```python
from build123d import *

# Parameters (mm, degrees)
SKETCH1_W           = 42.2
SKETCH1_H           = 5
SKETCH1_H_2         = 20
SKETCH1_R           = 1.275
SKETCH1_R_2         = 13
BOSS_EXTRUDE3_DEPTH = 5
SKETCH1_3_W         = 42.2
SKETCH1_3_H         = 5
BOSS_EXTRUDE4_DEPTH = 50
CUT_EXTRUDE1_DEPTH  = 109.583838576
SKETCH3_R           = 2.5
CUT_EXTRUDE2_DEPTH  = 81.037803568
SKETCH5_W           = 82.2
SKETCH5_H           = 50
SKETCH5_R           = 2.5
CUT_EXTRUDE3_DEPTH  = 2


with BuildPart() as part:
    # Sketch1 → Boss-Extrude3 (new body)
    # profile 1 of 6: a face of its own
    with BuildSketch(Plane(origin=(0, 0, 0), x_dir=(1, 0, 0), z_dir=(0, 1, 0))):
        with Locations((0, 43.6)):
            Rectangle(SKETCH1_W, SKETCH1_H)
    # profile 2 of 6: a face of its own
    with BuildSketch(Plane(origin=(0, 0, 0), x_dir=(1, 0, 0), z_dir=(0, 1, 0))):
        with Locations((0, 31.1)):
            Rectangle(SKETCH1_W, SKETCH1_H_2)
    # profile 3 of 6: a face of its own
    with BuildSketch(Plane(origin=(0, 0, 0), x_dir=(1, 0, 0), z_dir=(0, 1, 0))):
        Polygon((-21.1, -17.101), (-21.1, 17.101), (-21.1, 21.1), (-21.1, 41.1), (-21.1, 46.1), (-28.1, 46.1), (-28.1, -46.1), (-21.1, -46.1), (-21.1, -41.1), (-21.1, -21.1), align=None)
    # profile 4 of 6: a face of its own
    with BuildSketch(Plane(origin=(0, 0, 0), x_dir=(1, 0, 0), z_dir=(0, 1, 0))):
        Polygon((-21.1, 21.1), (-21.1, 17.101), (-21.1, -17.101), (-21.1, -21.1), (-17.101, -21.1), (17.101, -21.1), (21.1, -21.1), (21.1, -17.101), (21.1, 17.101), (21.1, 21.1), align=None)
        with Locations(Location((-15.5, -15.5, 0), (0, 0, 270))):
            Circle(SKETCH1_R, mode=Mode.SUBTRACT)
        with Locations(Location((15.5, -15.5, 0), (0, 0, 270))):
            Circle(SKETCH1_R, mode=Mode.SUBTRACT)
        with Locations(Location((-15.5, 15.5, 0), (0, 0, 270))):
            Circle(SKETCH1_R, mode=Mode.SUBTRACT)
        with Locations(Location((0, 0, 0), (0, 0, 270))):
            Circle(SKETCH1_R_2, mode=Mode.SUBTRACT)
        with Locations(Location((15.5, 15.5, 0), (0, 0, 270))):
            Circle(SKETCH1_R, mode=Mode.SUBTRACT)
    # profile 5 of 6: a face of its own
    with BuildSketch(Plane(origin=(0, 0, 0), x_dir=(1, 0, 0), z_dir=(0, 1, 0))):
        Polygon((-17.101, -21.1), (-21.1, -21.1), (-21.1, -41.1), (21.1, -41.1), (21.1, -21.1), (17.101, -21.1), align=None)
    # profile 6 of 6: a face of its own
    with BuildSketch(Plane(origin=(0, 0, 0), x_dir=(1, 0, 0), z_dir=(0, 1, 0))):
        with Locations((0, -43.6)):
            Rectangle(SKETCH1_W, SKETCH1_H)
    extrude(amount=BOSS_EXTRUDE3_DEPTH)

    # Sketch1_3 → Boss-Extrude4 (add)
    with BuildSketch(Plane(origin=(0, 0, 0), x_dir=(1, 0, 0), z_dir=(0, 1, 0))):
        Polygon((-21.1, -17.101), (-21.1, 17.101), (-21.1, 21.1), (-21.1, 41.1), (-21.1, 46.1), (-28.1, 46.1), (-28.1, -46.1), (-21.1, -46.1), (-21.1, -41.1), (-21.1, -21.1), align=None)
        with Locations((0, -43.6)):
            Rectangle(SKETCH1_3_W, SKETCH1_3_H)
        with Locations((0, 43.6)):
            Rectangle(SKETCH1_3_W, SKETCH1_3_H)
    extrude(amount=-BOSS_EXTRUDE4_DEPTH)

    # Sketch2 → Cut-Extrude1 (cut, through all)
    with BuildSketch(Plane.XY.offset(46.1)):
        Polygon((21.1, 0), (-21.1, -50), (21.1, -50), align=None)
    extrude(amount=-CUT_EXTRUDE1_DEPTH, mode=Mode.SUBTRACT)

    # Sketch3 → Cut-Extrude2 (cut, through all)
    with BuildSketch(Plane(origin=(-21.1, 0, 0), x_dir=(0, 0, -1), z_dir=(1, 0, 0))):
        with Locations((-33.1, -25)):
            Circle(SKETCH3_R)
        with Locations(Location((33.1, -25, 0), (0, 0, 180))):
            Circle(SKETCH3_R)
    extrude(amount=-CUT_EXTRUDE2_DEPTH, mode=Mode.SUBTRACT)

    # Sketch5 → Cut-Extrude3 (cut)
    with BuildSketch(Plane(origin=(-21.1, 0, 0), x_dir=(0, 0, -1), z_dir=(1, 0, 0))):
        with Locations((0, -25)):
            Rectangle(SKETCH5_W, SKETCH5_H)
        with Locations((33.1, -25)):
            Circle(SKETCH5_R, mode=Mode.SUBTRACT)
        with Locations((-33.1, -25)):
            Circle(SKETCH5_R, mode=Mode.SUBTRACT)
    extrude(amount=-CUT_EXTRUDE3_DEPTH, mode=Mode.SUBTRACT)


solid = part.part
```
Work out the finished part from the listing and answer in its coordinate system (mm). A direction names the side the tool comes from. Give positions to 0.01 mm unless a question says otherwise; leave off trailing zeros. Order: outer loops, then holes, each group sorted by start corner. A loop starts at its lowest first (then second) coordinate and runs counter-clockwise, first axis right, second up. Notation, with made-up numbers: (66, 71.25) - (73, 71.25) arc R20 ccw to (73, 84.25) - close; hole circle Ø5 at (3, 27.5). An arc over 180 degrees is marked (long way). One line per item, written item: value. Start each with the question number.
1. Consider line 1 (X direction, y = 2.2, z = 0); line 2 (Z direction, x = -4, y = -13); line 3 (Y direction, x = -26, z = 33). Determine where each line is inside the solid, lowest interval first.
2. Section C-C, the plane y = -25 is taken. Write down the section's boundary in (x, z).
3. Section B-B, the plane x = 0 is taken. Write down the section's boundary in (y, z), then the cut area to 3 significant figures.
4. Section A-A, the plane z = -15.5 is taken. Write down the section's boundary in (x, y) (3 decimals).
5. Section D-D, the plane z = -33.1 is taken. Write down the section's boundary in (x, y), then the cut area to 3 significant figures.
6. Which of the six approach directions +Z, -Z, +X, -X, +Y, -Y give full straight-line access (tool end or side, diameter ignored) to faces 4 (the face through (-25.56, -27.11, -31.76)), 5 (the face through (-11, -20, 41.1))?
7. Each of these flat-tipped pins is pushed along its axis until it touches: pin 1 Ø3 at (x, z) = (8.5, -35) entering from -Y; pin 2 Ø15 at (y, z) = (-14.5, 11) entering from +X; pin 3 Ø3.5 at (x, z) = (-15.5, -15.5) entering from +Y. Where does it stop, or does it pass through?
8. For a pull along Z with two mould halves and no side action, classify faces 1 (the face through (-14.64, 2.46, 14.56)), 2 (the face through (0, -25, -44)), 3 (the face through (-9, -16, 46.1)) as released by +Z, released by -Z, zero draft, split by the parting line, or undercut.
Filled sheet:
1. line 1: -28.1 to -13, 13 to 21.1
1. line 2: -46.1 to -41.1, 41.1 to 46.1
1. line 3: -50 to -27.5, -22.5 to 5
2. outline: (-28.1, -46.1) - (0, -46.1) - (0, -41.1) - (-23.1, -41.1) - (-23.1, -35.6) - (-28.1, -35.6) - close; (-28.1, -30.6) - (-23.1, -30.6) - (-23.1, 30.6) - (-28.1, 30.6) - close; (-28.1, 35.6) - (-23.1, 35.6) - (-23.1, 41.1) - (0, 41.1) - (0, 46.1) - (-28.1, 46.1) - close
3. outline: (-25, -46.1) - (5, -46.1) - (5, -13) - (0, -13) - (0, -41.1) - (-25, -41.1) - close; (-25, 41.1) - (0, 41.1) - (0, 13) - (5, 13) - (5, 46.1) - (-25, 46.1) - close
3. area: 581 mm²
4. outline: (-28.1, -50) - (-23.1, -50) - (-23.1, 0) - (-16.775, 0) - (-16.775, 5) - (-28.1, 5) - close; (-14.225, 0) - (14.225, 0) - (14.225, 5) - (-14.225, 5) - close; (16.775, 0) - (21.1, 0) - (21.1, 5) - (16.775, 5) - close
5. outline: (-28.1, -50) - (-23.1, -50) - (-23.1, -27.5) - (-28.1, -27.5) - close; (-28.1, -22.5) - (-23.1, -22.5) - (-23.1, 0) - (21.1, 0) - (21.1, 5) - (-28.1, 5) - close
5. area: 471 mm²
6. face 4: +X, -X
6. face 5: +X, -Y
7. pin 1: y = 0
7. pin 2: x = -23.1
7. pin 3: y = 5
8. face 1: undercut
8. face 2: zero draft
8. face 3: released by +Z
